Build history of the part. All positions in model axes, mm. A direction names the side the tool comes from. Coordinates: 2 decimals unless noted, no trailing zeros. Write each loop counter-clockwise with the first axis right and the second up, starting at its lowest first coordinate (ties: lowest second). Pieces come first, ordered by that corner, then holes.
```python
from build123d import *

# Parameters (mm, degrees)
SKETCH1_R           = 1.6
BOSS_EXTRUDE1_DEPTH = 0.4


with BuildPart() as part:
    # Sketch1 → Boss-Extrude1 (new body)
    with BuildSketch(Plane(origin=(0, 0, 0), x_dir=(1, 0, 0), z_dir=(0, 1, 0))):
        with BuildLine():
            Line((29.237843605, 13.960963482), (24.049079653, -21.711788683))
            ThreePointArc((24.049079653, -21.711788683), (17.208573183, -27.452231403), (9.060814288, -31.107260317))
            Line((9.060814288, -31.107260317), (-9.060814288, -31.107260317))
            ThreePointArc((-9.060814288, -31.107260317), (-24.689356555, 20.980840614), (29.237843605, 13.960963482))
        make_face()
        with Locations(Location((-17.5, 23, 0), (0, 0, 270))):
            Circle(SKETCH1_R, mode=Mode.SUBTRACT)
        with Locations(Location((-17.5, -23, 0), (0, 0, 270))):
            Circle(SKETCH1_R, mode=Mode.SUBTRACT)
        with Locations(Location((17.5, -23, 0), (0, 0, 270))):
            Circle(SKETCH1_R, mode=Mode.SUBTRACT)
        with Locations(Location((17.5, 23, 0), (0, 0, 270))):
            Circle(SKETCH1_R, mode=Mode.SUBTRACT)
        with BuildLine():
            Line((-4, -24.107260317), (4, -24.107260317))
            ThreePointArc((4, -24.107260317), (8.793181532, -28.027829543), (11.685431528, -22.552398764))
            ThreePointArc((11.685431528, -22.552398764), (12.499954018, -22.111335318), (13.297853098, -21.640866502))
            ThreePointArc((13.297853098, -21.640866502), (21.8608918, -17.056148201), (24.225281505, -7.63516444))
            ThreePointArc((24.225281505, -7.63516444), (25.005340406, -4.460151477), (25.371103528, -1.211241423))
            ThreePointArc((25.371103528, -1.211241423), (25.13782952, 13.24356348), (13.348031622, 21.609952611))
            ThreePointArc((13.348031622, 21.609952611), (0, 25.4), (-13.348031622, 21.609952611))
            ThreePointArc((-13.348031622, 21.609952611), (-25.13782952, 13.24356348), (-25.371103528, -1.211241423))
            ThreePointArc((-25.371103528, -1.211241423), (-25.005340406, -4.460151477), (-24.225281505, -7.63516444))
            ThreePointArc((-24.225281505, -7.63516444), (-21.8608918, -17.056148201), (-13.297853098, -21.640866502))
            ThreePointArc((-13.297853098, -21.640866502), (-12.499954018, -22.111335318), (-11.685431528, -22.552398764))
            ThreePointArc((-11.685431528, -22.552398764), (-8.793181532, -28.027829543), (-4, -24.107260317))
        make_face(mode=Mode.SUBTRACT)
    extrude(amount=BOSS_EXTRUDE1_DEPTH)


solid = part.part
```
1. Flat gauge pin, fed straight in: pin 1 (5 mm diameter, centred on x = 17.5, z = -23, fed in from -Y). Where does the tip first touch, or does it go through?
Computed values:
pin 1: stops at y = 0
2. Saw through at D-D on x = -17.5. List the corners of the cut face in (y, z), plus the area to 3 significant figures.
Computed values:
outline: (0, -27.27) - (0.4, -27.27) - (0.4, -24.6) - (0, -24.6) - close; (0, -21.4) - (0.4, -21.4) - (0.4, -20.4) - (0, -20.4) - close; (0, 20.54) - (0.4, 20.54) - (0.4, 21.4) - (0, 21.4) - close; (0, 24.6) - (0.4, 24.6) - (0.4, 27.27) - (0, 27.27) - close
area: 2.88 mm2
3. 3-axis set-ups, long thin cutter, end or side, ignore diameter. For faces 1 (the face through (-13, 0, -22)), 2 (the face through (-21.946, 0.197, 16.945)): which of +Z, -Z, +X, -X, +Y, -Y reach the whole face in a straight line?
Computed values:
face 1: +Z, -Z, +X, -X, -Y
face 2: +Y, -Y
4. Mould opens along Z. For faces 3 (the face through (-25.04, 0.2, -13.43)), 4 (the face through (-25.265, 0.197, -20.284)), 5 (the face through (26.68, 0.2, 3.63)) say: +Z half, -Z half, draft (parallel to the pull), parting line (faces both ways), or undercut.
Computed values:
face 3: undercut
face 4: parting line
face 5: +Z half
5. Saw through at A-A on x = 0. List the corners of the cut face in (y, z).
Computed values:
outline: (0, -32.4) - (0.4, -32.4) - (0.4, -25.4) - (0, -25.4) - close; (0, 24.11) - (0.4, 24.11) - (0.4, 31.11) - (0, 31.11) - close
6. Probe line 1 along X through (y, z) = (0.1, 23); line 2 along Z through (x, y) = (5.5, 0.05); line 3 along X through (y, z) = (0.35, -23). List the from-to ranges inside material, lowest first.
Computed values:
line 1: x = -22.82 to -19.1, -15.9 to -11.84, 11.84 to 15.9, 19.1 to 22.82
line 2: z = -31.93 to -24.8, 27.23 to 31.11
line 3: x = -22.82 to -19.1, -15.9 to -10.78, 10.78 to 15.9, 19.1 to 22.82
7. Saw through at B-B on y = 0.1. List the corners of the cut face in (x, z).
Computed values:
outline: (-9.06, 31.11) arc R32.4 ccw (long way) to (29.24, -13.96) - (24.05, 21.71) arc R32.4 ccw to (9.06, 31.11) - close; hole (-25.37, 1.21) arc R16 ccw to (-13.35, -21.61) arc R25.4 ccw to (13.35, -21.61) arc R16 ccw to (25.37, 1.21) arc R25.4 ccw to (24.23, 7.64) arc R12 ccw to (13.3, 21.64) arc R25.4 ccw to (11.69, 22.55) arc R4 ccw (long way) to (4, 24.11) - (-4, 24.11) arc R4 ccw (long way) to (-11.69, 22.55) arc R25.4 ccw to (-13.3, 21.64) arc R12 ccw to (-24.23, 7.64) arc R25.4 ccw to start; hole circle Ø3.2 at (-17.5, -23); hole circle Ø3.2 at (-17.5, 23); hole circle Ø3.2 at (17.5, -23); hole circle Ø3.2 at (17.5, 23)
8. Saw through at C-C on z = -23. List the corners of the cut face in (x, y).
Computed values:
outline: (-22.82, 0) - (-19.1, 0) - (-19.1, 0.4) - (-22.82, 0.4) - close; (-15.9, 0) - (-10.78, 0) - (-10.78, 0.4) - (-15.9, 0.4) - close; (10.78, 0) - (15.9, 0) - (15.9, 0.4) - (10.78, 0.4) - close; (19.1, 0) - (22.82, 0) - (22.82, 0.4) - (19.1, 0.4) - close
